```python
from build123d import *

# Parameters (mm, degrees)
BOSS_EXTRUDE1_DEPTH = 2
SKETCH2_R           = 1.5
CUT_EXTRUDE1_DEPTH  = 1


with BuildPart() as part:
    # Sketch1 → Boss-Extrude1 (new body)
    with BuildSketch(Plane(origin=(0, 0, 0), x_dir=(1, 0, 0), z_dir=(0, 1, 0))):
        Polygon((0, 6.651075101), (-3.84, 0), (0, -6.651075101), (3.84, 0), align=None)
    extrude(amount=BOSS_EXTRUDE1_DEPTH)

    # Sketch2 → Cut-Extrude1 (cut)
    with BuildSketch(Plane(origin=(0, 0, 0), x_dir=(-1, 0, 0), z_dir=(0, -1, 0))):
        Circle(SKETCH2_R)
    extrude(amount=-CUT_EXTRUDE1_DEPTH, mode=Mode.SUBTRACT)


solid = part.part
```
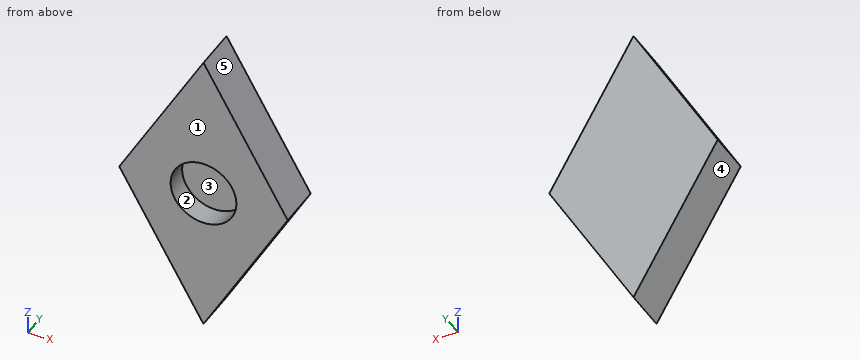
Check sheet for the modelled part. Datum: model origin and axes. Units: mm. Face numbers are marked on the shaded views. A direction names the side the tool comes from. Coordinates: 2 decimals unless noted, no trailing zeros. Order: outer loops, then holes, each group sorted by start corner. A loop starts at its lowest first (then second) coordinate and runs counter-clockwise, first axis right, second up. Notation, with made-up numbers: M 12,-24.75 L 26,-24.75 A11 cw 26,-10.75 Z; hole C 6.25,62.25 d3. An arc over 180 degrees is marked long. Write each question's results on one line, items separated by ' | '. Start each with the question number.
1. Cross-section at A-A on y = 0.6. Record the cut outline in (x, z).
2. Mould release check, pull along Z, two halves, no side actions. Record for the marked faces 3, 4 and 5: +Z half, -Z half, draft (parallel to the pull), parting line (faces both ways), or undercut.
3. Cross-section at C-C on y = 1.45. Record the cut outline in (x, z).
4. Go/stop test with flat-tipped pins: P1, Ø1, axis at y = 1, z = 3, coming from the +X side; P2, Ø1, axis at x = -3, y = 0.5, coming from the -Z side; P3, Ø0.9, axis at x = 0.5, z = -0.5, coming from the -Y side. Record where each tip stops, or that it passes through.
5. Cross-section at B-B on x = 0.25. Record the cut outline in (y, z), and give its area (3 significant figures).
6. Material ranges on probe 1 along Y at (x, z) = (-0.5, -1); probe 2 along Z at (x, y) = (-1, 0.85); probe 3 along X at (y, z) = (0.15, 6.25), recorded low to high.
7. Cross-section at D-D on z = 4.5. Record the cut outline in (x, y), and give its area (3 significant figures).
8. Access from +Z, -Z, +X, -X, +Y, -Y to the whole of each face (thin tool, end or side, straight path). Record for the marked faces 1 and 2.
Checks:
1) outline: M -3.84,0 L 0,-6.65 L 3.84,0 L 0,6.65 Z; hole C 0,0 d3
2) face 3: undercut | face 4: -Z half | face 5: +Z half
3) outline: M -3.84,0 L 0,-6.65 L 3.84,0 L 0,6.65 Z
4) P1: stops at x = 2.4 | P2: stops at z = -2.32 | P3: stops at y = 1
5) outline: M 0,-6.22 L 2,-6.22 L 2,6.22 L 0,6.22 L 0,1.48 L 1,1.48 L 1,-1.48 L 0,-1.48 Z | area: 21.9 mm²
6) probe 1: y = 1 to 2 | probe 2: z = -4.92 to -1.12, 1.12 to 4.92 | probe 3: x = -0.23 to 0.23
7) outline: M -1.24,0 L 1.24,0 L 1.24,2 L -1.24,2 Z | area: 4.97 mm²
8) face 1: +Z, -Z, +X, -X, -Y | face 2: -Y
